Input: dimensioned drawing with shaded views. Units: mm. Origin: part minimum x, y, z. Round coordinates to 2 decimals unless told otherwise and drop trailing zeros. Loops run counter-clockwise (first coordinate to the right, second up) from the corner with the lowest first, then second, coordinate; pieces in that order, holes last.
1) Section C-C, the plane y = 6.5. Return loops of the section in (x, z).
2) Section B-B, the plane z = 30. Return loops of the section in (x, y).
3) Section A-A, the plane x = 30. Return loops of the section in (y, z), and give its area (3 significant figures).
4) First-contact query: pin 1 (5 mm diameter, centred on x = 17.5, y = 8.5, fed in from -Z); pin 2 (1 mm diameter, centred on y = 6, z = 49, fed in from +X); pin 3 (4 mm diameter, centred on x = 25.5, y = 5, fed in from -Z). Flat tips, straight axial feed; report the tip coordinate or a pass-through.
5) Ray query, line 1 along X through (y, z) = (7.5, 30); line 2 along Z through (x, y) = (30.5, 7.5); line 3 along Z through (x, y) = (31, 6.5). Return the intervals inside material, ascending.
6) Draft query along Z for the marked faces 1, 2 and 3. Return one class per face: pulls with the +Z half, pulls with the -Z half, needs draft (parallel to the pull), parting line crosses it, or undercut.
7) Section D-D, the plane x = 9. Return loops of the section in (y, z).
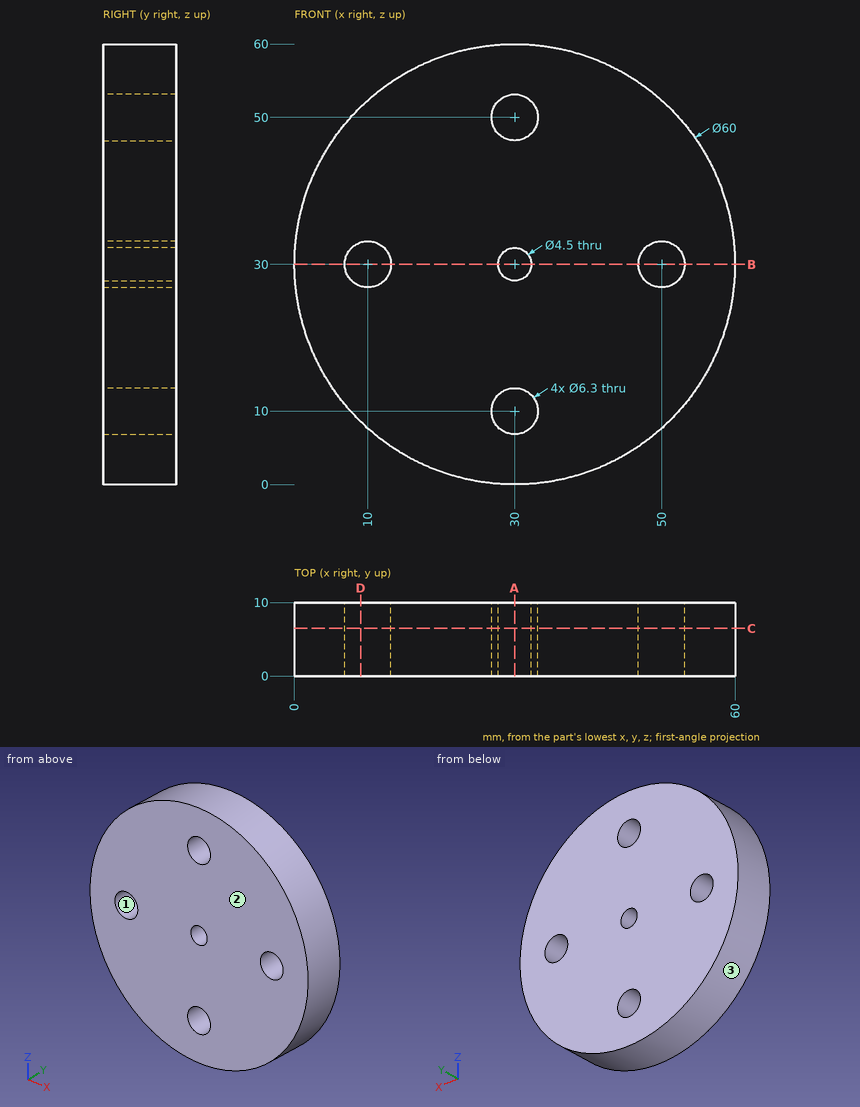
Final values:
1. outline: circle Ø60 at (30, 30); hole circle Ø6.3 at (10, 30); hole circle Ø6.3 at (30, 10); hole circle Ø6.3 at (30, 50); hole circle Ø4.5 at (30, 30); hole circle Ø6.3 at (50, 30)
2. outline: (0, 0) - (6.85, 0) - (6.85, 10) - (0, 10) - close; (13.15, 0) - (27.75, 0) - (27.75, 10) - (13.15, 10) - close; (32.25, 0) - (46.85, 0) - (46.85, 10) - (32.25, 10) - close; (53.15, 0) - (60, 0) - (60, 10) - (53.15, 10) - close
3. outline: (0, 0) - (10, 0) - (10, 6.85) - (0, 6.85) - close; (0, 13.15) - (10, 13.15) - (10, 27.75) - (0, 27.75) - close; (0, 32.25) - (10, 32.25) - (10, 46.85) - (0, 46.85) - close; (0, 53.15) - (10, 53.15) - (10, 60) - (0, 60) - close
3. area: 429 mm2
4. pin 1: stops at z = 1.72
4. pin 2: stops at x = 53.62
4. pin 3: stops at z = 0.1
5. line 1: x = 0 to 6.85, 13.15 to 27.75, 32.25 to 46.85, 53.15 to 60
5. line 2: z = 0 to 6.89, 13.11 to 27.81, 32.19 to 46.89, 53.11 to 60
5. line 3: z = 0.02 to 7.01, 12.99 to 27.98, 32.02 to 47.01, 52.99 to 59.98
6. face 1: undercut
6. face 2: needs draft
6. face 3: parting line crosses it
7. outline: (0, 8.58) - (10, 8.58) - (10, 27.01) - (0, 27.01) - close; (0, 32.99) - (10, 32.99) - (10, 51.42) - (0, 51.42) - close
